from build123d import *

# Parameters (mm, degrees)
BOSS_EXTRUDE1_DEPTH = 203.2
CUT_EXTRUDE1_DEPTH  = 201.422
CUT_EXTRUDE2_DEPTH  = 101.6


with BuildPart() as part:
    # Sketch2 → Boss-Extrude1 (new body)
    with BuildSketch(Plane.XY):
        with BuildLine():
            Line((-69.85, 0), (69.85, 0))
            ThreePointArc((69.85, 0), (0, 69.85), (-69.85, 0))
        make_face()
    extrude(amount=BOSS_EXTRUDE1_DEPTH)

    # Sketch3 → Cut-Extrude1 (cut)
    with BuildSketch(Plane.XY.offset(203.2)):
        with BuildLine():
            Line((-62.585749472, 1.778), (62.585749472, 1.778))
            ThreePointArc((62.585749472, 1.778), (0, 62.611), (-62.585749472, 1.778))
        make_face()
    extrude(amount=-CUT_EXTRUDE1_DEPTH, mode=Mode.SUBTRACT)

    # Sketch5 → Cut-Extrude2 (cut)
    with BuildSketch(Plane.XY.offset(203.2)):
        with BuildLine():
            Line((66.363298263, 0), (63.823298263, 0))
            ThreePointArc((63.823298263, 0), (-0.946701737, 64.77), (-65.716701737, 0))
            Line((-65.716701737, 0), (-68.256701737, 0))
            ThreePointArc((-68.256701737, 0), (-0.946701737, 67.31), (66.363298263, 0))
        make_face()
    extrude(amount=-CUT_EXTRUDE2_DEPTH, mode=Mode.SUBTRACT)


solid = part.part
Geometry check sheet. Reference: the model listing, model coordinates, mm. A direction names the side the tool comes from. Round coordinates to 2 decimals unless told otherwise and drop trailing zeros. Order: outer loops, then holes, each group sorted by start corner. A loop starts at its lowest first (then second) coordinate and runs counter-clockwise, first axis right, second up. Notation, with made-up numbers: (-19.75, -10.75) - (28.25, -10.75) arc R20 cw to (28.25, 6.25) - close; hole circle Ø5 at (7, 9). An arc over 180 degrees is marked (long way). One line per question, with ' | ' between items. Start each with the question number.
(1) Sectioned sample at B-B on x = 35.5. Record the cut outline in (y, z), and give its area (3 significant figures).
(2) Release check for a two-part mould opening along X. For faces 1 (the flat face through (-1, 0, 100)), 2 (the flat face through (-1, 26, 1.778)), 3 (the cylindrical face through (1.536, 69.833, 100.178)) record: released by +X, released by -X, zero draft, split by the parting line, or undercut.
(3) Thickness scan on L1, parallel to Y at x = 56, z = 118; L2, parallel to X at y = 4.5, z = 168.5; L3, parallel to Y at x = -10.5, z = 141. Record the ranges inside material, lowest first. Write a range as [from, to].
(4) Depth check by flat-ended pin: pin 1 Ø5 at (x, z) = (27, 77.5) entering from +Y; pin 2 Ø6 at (x, y) = (2.5, 8) entering from +Z; pin 3 Ø3 at (x, z) = (9.5, 34.5) entering from +Y. Enter the tip coordinate at first touch or a pass-through.
(5) Access from +Z, -Z, +X, -X, +Y, -Y to the whole of each face (thin tool, end or side, straight path). Record for faces 4 (the flat face through (26, 64, 203.2)), 5 (the cylindrical face through (0.478, 64.754, 153.111)).
(6) Sectioned sample at C-C on y = 16. Record the cut outline in (x, z).
Conclusion:
1) outline: (0, 0) - (60.16, 0) - (60.16, 203.2) - (56.59, 203.2) - (56.59, 101.6) - (53.54, 101.6) - (53.54, 203.2) - (51.57, 203.2) - (51.57, 1.78) - (1.78, 1.78) - (1.78, 203.2) - (0, 203.2) - close | area: 1,880 mm2
2) face 1: zero draft | face 2: undercut | face 3: split by the parting line
3) L1: y = [0, 1.78], [28, 30.86], [35.88, 41.75] | L2: x = [-69.7, -68.11], [-65.56, -62.45], [62.45, 63.67], [66.21, 69.7] | L3: y = [0, 1.78], [61.72, 64.06], [66.63, 69.06]
4) pin 1: stops at y = 65.41 | pin 2: stops at z = 1.78 | pin 3: stops at y = 69.39
5) face 4: +Z, +X, -X, +Y, -Y | face 5: +Z
6) outline: (-67.99, 0) - (67.99, 0) - (67.99, 203.2) - (64.43, 203.2) - (64.43, 101.6) - (61.82, 101.6) - (61.82, 203.2) - (60.53, 203.2) - (60.53, 1.78) - (-60.53, 1.78) - (-60.53, 203.2) - (-63.71, 203.2) - (-63.71, 101.6) - (-66.33, 101.6) - (-66.33, 203.2) - (-67.99, 203.2) - close
